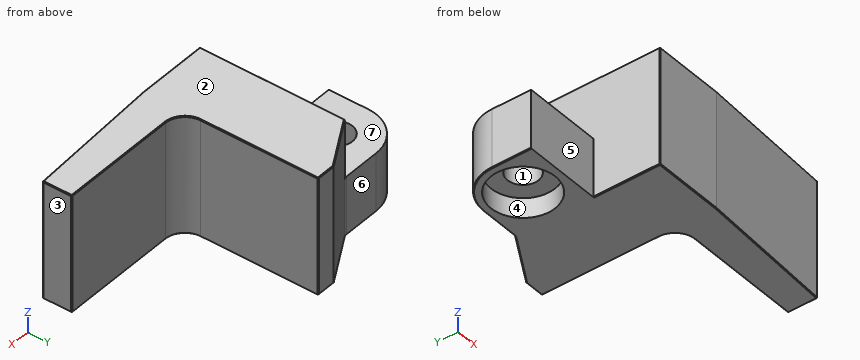
```python
from build123d import *
from OCP.BRepFilletAPI import BRepFilletAPI_MakeChamfer

# Parameters (mm, degrees)
BOSS_EXTRUDE1_DEPTH                                  = 38.1
FILLET2_R                                            = 6.35
CUT_EXTRUDE1_START                                   = -19.05
CUT_EXTRUDE1_DEPTH                                   = 19.05
FILLET3_R                                            = 2.54
CBORE_FOR_3_8_BINDING_HEAD_MACHINE_SCREW_D           = 10.0838
CBORE_FOR_3_8_BINDING_HEAD_MACHINE_SCREW_CBORE_D     = 20.828
CBORE_FOR_3_8_BINDING_HEAD_MACHINE_SCREW_CBORE_DEPTH = 6.4262
CHAMFER3_SIZE                                        = 0.254
CHAMFER5_SIZE                                        = 0.254
CHAMFER5_SIZE2                                       = 0.270375256


with BuildPart() as part:
    # Sketch1 → Boss-Extrude1 (new body)
    with BuildSketch(Plane.XY):
        with BuildLine():
            Line((0, 0), (44.45, 0))
            Line((44.45, 0), (44.45, -9.525))
            Line((44.45, -9.525), (0, -12.1446544))
            Line((0, -12.1446544), (-22.9902, -12.1446544))
            Line((-22.9902, -12.1446544), (-22.9902, 9.4453456))
            Line((-22.9902, 9.4453456), (-48.3902, 9.4453456))
            Line((-48.3902, 9.4453456), (-48.3902, 22.1453456))
            ThreePointArc((-48.3902, 22.1453456), (-44.670456121, 31.125601721), (-35.6902, 34.8453456))
            Line((-35.6902, 34.8453456), (-22.9902, 34.8453456))
            Line((-22.9902, 34.8453456), (-6.35, 44.45))
            Line((-6.35, 44.45), (0, 44.45))
            Line((0, 44.45), (0, 0))
        make_face()
    extrude(amount=BOSS_EXTRUDE1_DEPTH)

    # Fillet2
    fillet2_edges = [part.edges().sort_by_distance(p)[0] for p in [
        (0, 0, 19.05),
    ]]
    fillet(fillet2_edges, radius=FILLET2_R)

    # Sketch3 → Cut-Extrude1 (cut)
    with BuildSketch(Plane.XY.offset(38.1).offset(CUT_EXTRUDE1_START)):
        with BuildLine():
            Line((-48.3902, 9.4453456), (-22.9902, 9.4453456))
            Line((-22.9902, 9.4453456), (-22.9902, 34.8453456))
            Line((-22.9902, 34.8453456), (-35.6902, 34.8453456))
            ThreePointArc((-35.6902, 34.8453456), (-44.670456121, 31.125601721), (-48.3902, 22.1453456))
            Line((-48.3902, 22.1453456), (-48.3902, 9.4453456))
        make_face()
    extrude(amount=CUT_EXTRUDE1_DEPTH, mode=Mode.SUBTRACT)

    # Fillet3
    fillet3_edges = [part.edges().sort_by_distance(p)[0] for p in [
        (-22.9902, 34.8453456, 9.525),
    ]]
    fillet(fillet3_edges, radius=FILLET3_R)

    # CBORE for 3/8 Binding Head Machine Screw1 (through all)
    with Locations(Plane(origin=(0, 0, 0), x_dir=(-1, 0, 0), z_dir=(0, 0, -1))):
        with Locations((35.6902, 22.1453456)):
            CounterBoreHole(CBORE_FOR_3_8_BINDING_HEAD_MACHINE_SCREW_D / 2, CBORE_FOR_3_8_BINDING_HEAD_MACHINE_SCREW_CBORE_D / 2, CBORE_FOR_3_8_BINDING_HEAD_MACHINE_SCREW_CBORE_DEPTH)

    # Chamfer3
    chamfer3_edges = [part.edges().sort_by_distance(p)[0] for p in [
        (25.4, 0, 0),
        (44.45, 0, 19.05),
        (0, 44.45, 19.05),
        (0, 25.4, 0),
        (0, 25.4, 38.1),
        (1.859871939, 1.859871939, 0),
        (1.859871939, 1.859871939, 38.1),
        (25.4, 0, 38.1),
    ]]
    chamfer(chamfer3_edges, length=CHAMFER3_SIZE)

    # Chamfer5: one chamfer whose edges measure the first distance from different faces: ONE call of the kernel's chamfer builder (chamfer() names one face for all edges)
    chamfer5_edges_1 = [part.edges().sort_by_distance(p)[0] for p in [
        (44.45, -4.8895, 0),
        (-14.6701, 39.6476728, 38.1),
        (-48.3902, 15.7953456, 0),
        (-44.670456121, 31.125601721, 0),
        (-14.375444039, 39.817746998, 0),
        (44.45, -4.8895, 38.1),
        (-29.680416649, 34.8453456, 0),
        (-23.013375005, 34.931855935, 0),
        (-3.302, 44.45, 38.1),
        (-3.302, 44.45, 0),
    ]]
    chamfer5_edges_2 = [part.edges().sort_by_distance(p)[0] for p in [
        (44.45, -9.525, 19.05),
    ]]
    chamfer5_side_2 = [part.faces().sort_by_distance(p)[0] for p in [
        (22.225, -10.8348272, 19.05),
    ]]
    chamfer5 = BRepFilletAPI_MakeChamfer(part.part.solid().wrapped)
    for e in chamfer5_edges_1:
        chamfer5.Add(CHAMFER5_SIZE, e.wrapped)
    for e in chamfer5_edges_2:
        chamfer5.Add(CHAMFER5_SIZE, CHAMFER5_SIZE2, e.wrapped, chamfer5_side_2[0].wrapped)  # the first distance lies on this face
    add(Compound.cast(chamfer5.Shape()), mode=Mode.REPLACE)

    # Chamfer6
    # the kernel refuses this chamfer: 0.693641083, 0.254 mm, written as the material it takes off along each edge
    with BuildSketch(Plane(origin=(-22.820866667, -11.975321067, 0.169333333), x_dir=(0, -0.7071067811865468, 0.7071067811865481), z_dir=(-0.5773502691896234, -0.5773502691896274, -0.5773502691896264))) as chamfer6_piece_1:
        Polygon((-0.179605122, -0.103695066), (0.179605122, -0.103695066), (0, 0.207390132), align=None)
    extrude(amount=0.32262333, mode=Mode.SUBTRACT)
    with BuildSketch(Plane(origin=(-22.820866667, -11.975321067, 37.930666667), x_dir=(0, -0.70710678118655, -0.707106781186545), z_dir=(-0.5773502691896217, -0.5773502691896258, 0.5773502691896298))) as chamfer6_piece_2:
        Polygon((-0.179605122, 0.103695066), (0.179605122, 0.103695066), (0, -0.207390132), align=None)
    extrude(amount=0.32262333, mode=Mode.SUBTRACT)
    with BuildSketch(Plane(origin=(-22.9902, 34.8453456, 19.05), x_dir=(-0.009971465906807519, -0.9999502836979793, 0), z_dir=(0, 0, 1))) as chamfer6_piece_3:
        with BuildLine():
            Line((0.720476303, 0), (-0.15603149, 0.22562472))
            Line((-0.15603149, 0.22562472), (-0.16797676, 0.218570238))
            ThreePointArc((-0.16797676, 0.218570238), (-0.081514433, 0.11074615), (-0.01194527, -0.007054482))
            Line((-0.01194527, -0.007054482), (0.000138332, -0.013872132))
            ThreePointArc((0.000138332, -0.013872132), (0.360340666, -0.010280208), (0.720614636, -0.013872132))
            Line((0.720614636, -0.013872132), (0.720476303, 0))
        make_face()
    extrude(amount=20.597190759, mode=Mode.SUBTRACT)
    with BuildSketch(Plane(origin=(-22.9902, -12.797861879, 0), x_dir=(0.9996219169112968, 0, -0.027495876610586136), z_dir=(0, 1, 0))) as chamfer6_piece_4:
        with BuildLine():
            Line((0.261282992, 0), (-0.014362977, -0.26088792))
            Line((-0.014362977, -0.26088792), (-0.019441057, -0.260748241))
            ThreePointArc((-0.019441057, -0.260748241), (-0.008668824, -0.130403049), (-0.005078079, 0.000139679))
            Line((-0.005078079, 0.000139679), (0.000139679, 0.005078079))
            ThreePointArc((0.000139679, 0.005078079), (0.130682407, 0.001487335), (0.261422671, 0.005078079))
            Line((0.261422671, 0.005078079), (0.261282992, 0))
        make_face()
    extrude(amount=22.243207479, mode=Mode.SUBTRACT)
    with BuildSketch(Plane(origin=(44.848076027, -9.501539446, 0), x_dir=(-0.058810529584687465, 0.9978904240343144, -0.027495876610586504), z_dir=(-0.9982678522272378, -0.05883277326131908, 0)), Plane(origin=(44.848076027, -9.501539446, 38.1), x_dir=(0.0016176586742518812, -0.02744824968915599, -0.9996219169112968), z_dir=(-0.9982678522272378, -0.05883277326131908, 0))) as chamfer6_piece_5:
        with BuildLine():
            Line((0.261282992, 0), (-0.014362977, -0.26088792))
            Line((-0.014362977, -0.26088792), (-0.019441057, -0.260748241))
            ThreePointArc((-0.019441057, -0.260748241), (-0.008668824, -0.130403049), (-0.005078079, 0.000139679))
            Line((-0.005078079, 0.000139679), (0.000139679, 0.005078079))
            ThreePointArc((0.000139679, 0.005078079), (0.130682407, 0.001487335), (0.261422671, 0.005078079))
            Line((0.261422671, 0.005078079), (0.261282992, 0))
        make_face()
    extrude(amount=45.579101794, mode=Mode.SUBTRACT)
    with BuildSketch(Plane(origin=(0.653207479, -12.1446544, 0), x_dir=(0, 0.9996219169112968, -0.0274958766105868), z_dir=(-1, 0, 0)), Plane(origin=(0.653207479, -12.1446544, 38.1), x_dir=(0, -0.027495876610587867, -0.9996219169112968), z_dir=(-1, 0, 0))) as chamfer6_piece_6:
        with BuildLine():
            Line((0.261282992, 0), (-0.014362977, -0.26088792))
            Line((-0.014362977, -0.26088792), (-0.019441057, -0.260748241))
            ThreePointArc((-0.019441057, -0.260748241), (-0.008668824, -0.130403049), (-0.005078079, 0.000139679))
            Line((-0.005078079, 0.000139679), (0.000139679, 0.005078079))
            ThreePointArc((0.000139679, 0.005078079), (0.130682407, 0.001487335), (0.261422671, 0.005078079))
            Line((0.261422671, 0.005078079), (0.261282992, 0))
        make_face()
    extrude(amount=24.296614958, mode=Mode.SUBTRACT)
    with BuildSketch(Plane(origin=(-22.9902, -12.1446544, -0.653207479), x_dir=(0.9996219169112968, -0.027495876610587118, 0), z_dir=(0, 0, 1))) as chamfer6_piece_7:
        with BuildLine():
            Line((0.261282992, 0), (-0.014362977, 0.26088792))
            Line((-0.014362977, 0.26088792), (-0.019441057, 0.260748241))
            ThreePointArc((-0.019441057, 0.260748241), (-0.008668824, 0.130403049), (-0.005078079, -0.000139679))
            Line((-0.005078079, -0.000139679), (0.000139679, -0.005078079))
            ThreePointArc((0.000139679, -0.005078079), (0.130682407, -0.001487335), (0.261422671, -0.005078079))
            Line((0.261422671, -0.005078079), (0.261282992, 0))
        make_face()
    extrude(amount=39.406414958, mode=Mode.SUBTRACT)
    with BuildSketch(Plane(origin=(-22.9902, 35.205278751, 38.1), x_dir=(-0.027495876610587867, 0, -0.9996219169112968), z_dir=(0, -1, 0))) as chamfer6_piece_8:
        with BuildLine():
            Line((0.261282992, 0), (-0.014362977, 0.26088792))
            Line((-0.014362977, 0.26088792), (-0.019441057, 0.260748241))
            ThreePointArc((-0.019441057, 0.260748241), (-0.008668824, 0.130403049), (-0.005078079, -0.000139679))
            Line((-0.005078079, -0.000139679), (0.000139679, -0.005078079))
            ThreePointArc((0.000139679, -0.005078079), (0.130682407, -0.001487335), (0.261422671, -0.005078079))
            Line((0.261422671, -0.005078079), (0.261282992, 0))
        make_face()
    extrude(amount=48.00314063, mode=Mode.SUBTRACT)


solid = part.part
```
Verification items for the finished model (mm, model axes). Face numbers are marked on the shaded views. A direction names the side the tool comes from. Round coordinates to 2 decimals unless told otherwise and drop trailing zeros. Loops run counter-clockwise (first coordinate to the right, second up) from the corner with the lowest first, then second, coordinate; pieces in that order, holes last. Notation, with made-up numbers: (78.25, 4.25) -> (114.25, 4.25) arc R33 cw to (114.25, 35.25) -> close; hole circle Ø5 at (29.25, 23). An arc over 180 degrees is marked (long way). Answer as a JSON object with one key per item and string values.
Q1. Section check B-B (y = -2). Record the boundary of the cut face in (x, z), then the cut area to 3 significant figures.
Data:
{"outline": "(-22.99, 0.25) -> (-22.74, 0) -> (44.2, 0) -> (44.45, 0.25) -> (44.45, 37.85) -> (44.2, 38.1) -> (-22.74, 38.1) -> (-22.99, 37.85) -> close", "area": "2,570 mm2"}
Q2. Section check C-C (x = -33). Record the boundary of the cut face in (y, z), then the cut area to 3 significant figures.
Data:
{"outline": "(9.45, 0) -> (12.08, 0) -> (12.08, 6.43) -> (17.88, 6.43) -> (17.88, 19.05) -> (9.45, 19.05) -> close; (26.41, 6.43) -> (32.21, 6.43) -> (32.21, 0) -> (34.59, 0) -> (34.85, 0.25) -> (34.85, 19.05) -> (26.41, 19.05) -> close", "area": "247 mm2"}
Q3. Access from +Z, -Z, +X, -X, +Y, -Y to the whole of each face (thin tool, end or side, straight path). Record for the marked faces 5, 6 and 7.
Data:
{"face 5": "+Z, -Z, -X, -Y", "face 6": "+Z, -Z, -X, +Y", "face 7": "+Z, -X, +Y, -Y"}
Q4. Section check A-A (z = 16.5). Record the boundary of the cut face in (x, y).
Data:
{"outline": "(-48.39, 9.45) -> (-22.99, 9.45) -> (-22.99, -11.89) -> (-22.74, -12.14) -> (0, -12.14) -> (44.2, -9.54) -> (44.45, -9.25) -> (44.45, -0.25) -> (44.2, 0) -> (6.35, 0) arc R6.35 cw to (0, 6.35) -> (0, 44.2) -> (-0.25, 44.45) -> (-6.35, 44.45) -> (-22.4, 35.19) arc R2.54 cw to (-23.67, 34.85) -> (-35.69, 34.85) arc R12.7 ccw to (-48.39, 22.15) -> close; hole circle Ø10.08 at (-35.69, 22.15)"}
Q5. Draft check along X on the marked faces 1, 2, 3 and 4. Enter one of: pulls with the +X half, pulls with the -X half, needs draft (parallel to the pull), parting line crosses it, or undercut.
Data:
{"face 1": "undercut", "face 2": "needs draft", "face 3": "pulls with the +X half", "face 4": "undercut"}
Q6. Go/stop test with flat-tipped pins: P1, Ø12, axis at y = 8.5, z = 14, coming from the -X side; P2, Ø10.5, axis at x = -35, y = 18.5, coming from the -Z side; P3, Ø11.5, axis at y = 23.5, z = 12, coming from the +X side; P4, Ø5.5, axis at x = -32.5, z = 10.5, coming from the -Y side. Record where each tip stops, or that it passes through.
Data:
{"P1": "stops at x = -48.39", "P2": "stops at z = 6.43", "P3": "stops at x = 0", "P4": "stops at y = 9.45"}
Q7. Scan lines: line 1 (Y direction, x = -36, z = 17); line 2 (X direction, y = 22, z = 7.5); line 3 (X direction, y = -7, z = 35). Record each from-to range of solid material in increasing order. Write a range as from..to.
Data:
{"line 1": "y = 9.45..17.11, 27.18..34.84", "line 2": "x = -48.39..-40.73, -30.65..0", "line 3": "x = -22.99..44.45"}
Q8. Section check D-D (y = 19.5). Record the boundary of the cut face in (x, z).
Data:
{"outline": "(-48.39, 0.25) -> (-48.14, 0) -> (-45.76, 0) -> (-45.76, 6.43) -> (-39.98, 6.43) -> (-39.98, 19.05) -> (-48.39, 19.05) -> close; (-31.4, 6.43) -> (-25.62, 6.43) -> (-25.62, 0) -> (-0.25, 0) -> (0, 0.25) -> (0, 37.85) -> (-0.25, 38.1) -> (-22.74, 38.1) -> (-22.99, 37.85) -> (-22.99, 19.05) -> (-31.4, 19.05) -> close"}
